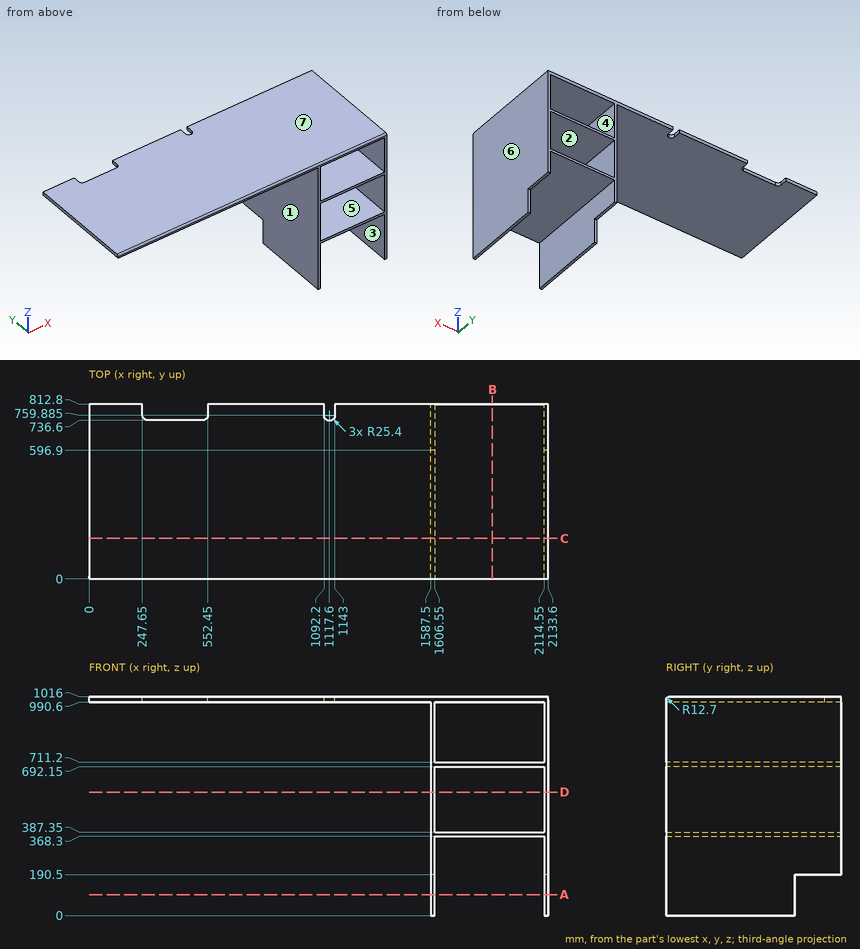
Geometry check sheet. Reference: drawing and pictorial views, mm from the part's lowest x, y, z. A direction names the side the tool comes from. Give positions to 0.01 mm unless a question says otherwise; leave off trailing zeros. Order: outer loops, then holes, each group sorted by start corner. A loop starts at its lowest first (then second) coordinate and runs counter-clockwise, first axis right, second up.
1. Section check C-C, the plane y = 188.5. Enter the section's corners in (x, z), and give its area (3 significant figures).
2. Release check for a two-part mould opening along X. For the marked faces 4, 5, 6 and 7 record: pulls with the +X half, pulls with the -X half, needs draft (parallel to the pull), parting line crosses it, or undercut.
3. Thickness scan on L1, parallel to Z at x = 2020, y = 701; L2, parallel to X at y = 732, z = 798; L3, parallel to Z at x = 586.5, y = 717. Record the ranges inside material, lowest first.
4. Gauge pin test, flat ends, axial feed: pin 1 Ø1.5 at (x, y) = (1152.5, 511) entering from -Z; pin 2 Ø10 at (y, z) = (395.5, 821) entering from -X; pin 3 Ø9.5 at (x, y) = (2123.5, 662) entering from -Z. Record the tip position at first contact, or that the pin passes through.
5. Section check D-D, the plane z = 573.5. Enter the section's corners in (x, y), and give its area (3 significant figures).
6. Section check A-A, the plane z = 97. Enter the section's corners in (x, y), and give its area (3 significant figures).
7. Access from +Z, -Z, +X, -X, +Y, -Y to the whole of each face (thin tool, end or side, straight path). Record for the marked faces 1, 2 and 3.
8. Section check B-B, the plane x = 1874.5. Enter the section's corners in (y, z).
Values follow:
1. outline: (0, 990.6) - (1587.5, 990.6) - (1587.5, 0) - (1606.55, 0) - (1606.55, 368.3) - (2114.55, 368.3) - (2114.55, 0) - (2133.6, 0) - (2133.6, 1016) - (0, 1016) - close; hole (1606.55, 387.35) - (2114.55, 387.35) - (2114.55, 692.15) - (1606.55, 692.15) - close; hole (1606.55, 711.2) - (2114.55, 711.2) - (2114.55, 990.6) - (1606.55, 990.6) - close
1. area: 111,000 mm2
2. face 4: undercut
2. face 5: undercut
2. face 6: pulls with the +X half
2. face 7: needs draft
3. L1: z = 368.3 to 387.35, 692.15 to 711.2, 990.6 to 1016
3. L2: x = 1587.5 to 1606.55, 2114.55 to 2133.6
3. L3: z = 990.6 to 1016
4. pin 1: stops at z = 990.6
4. pin 2: stops at x = 1587.5
4. pin 3: stops at z = 190.5
5. outline: (1587.5, 0) - (1606.55, 0) - (1606.55, 812.8) - (1587.5, 812.8) - close; (2114.55, 0) - (2133.6, 0) - (2133.6, 812.8) - (2114.55, 812.8) - close
5. area: 31,000 mm2
6. outline: (1587.5, 0) - (1606.55, 0) - (1606.55, 596.9) - (1587.5, 596.9) - close; (2114.55, 0) - (2133.6, 0) - (2133.6, 596.9) - (2114.55, 596.9) - close
6. area: 22,700 mm2
7. face 1: -Z, -X, +Y, -Y
7. face 2: +Y, -Y
7. face 3: -Z, +Y, -Y
8. outline: (0, 368.3) - (812.8, 368.3) - (812.8, 387.35) - (0, 387.35) - close; (0, 692.15) - (812.8, 692.15) - (812.8, 711.2) - (0, 711.2) - close; (0, 990.6) - (812.8, 990.6) - (812.8, 1016) - (12.7, 1016) arc R12.7 ccw to (0, 1003.3) - close
